Check sheet for the modelled part. Datum: model origin and axes. Units: mm. A direction names the side the tool comes from. Coordinates: 2 decimals unless noted, no trailing zeros. Loops run counter-clockwise (first coordinate to the right, second up) from the corner with the lowest first, then second, coordinate; pieces in that order, holes last. Notation, with made-up numbers: (9, 73.25) - (43, 73.25) arc R30 ccw to (43, 96.25) - close; hole circle Ø8 at (42, 73). An arc over 180 degrees is marked (long way). Use a Markdown table: item, result. Add a question column.
1) Tool access check on faces 4 (the flat face through (-9.5, -0.1, 19.2)), 5 (the cylindrical face through (-5.158, -3.955, 2.535)). Record the directions out of +Z, -Z, +X, -X, +Y, -Y that give a thin tool (end or side, any length) a straight path to the whole face; none if there is none.
2) Go/stop test with flat-tipped pins: P1, Ø6.5, axis at y = 1, z = 13.5, coming from the +X side; P2, Ø3.5, axis at x = 14, y = -6, coming from the -Z side. Record where each tip stops, or that it passes through.
3) Sectioned sample at A-A, the plane y = 6. Enter the section's corners in (x, z), then the cut area to 3 significant figures.
4) Draft check along Y on faces 1 (the cylindrical face through (-14, 0, 8)), 2 (the cylindrical face through (8.93, 0.13, 5.6)), 3 (the cylindrical face through (16.93, 8.9, 13.69)). Enter one of: pulls with the +Y half, pulls with the -Y half, needs draft (parallel to the pull), parting line crosses it, or undercut.
5) Sectioned sample at C-C, the plane x = 0. Enter the section's corners in (y, z), then the cut area to 3 significant figures.
6) Sectioned sample at B-B, the plane z = 18.5. Enter the section's corners in (x, y), then the cut area to 3 significant figures.
7) Thickness scan on line 1 (Y direction, x = 14, z = 20.75); line 2 (Y direction, x = -14, z = 10.5); line 3 (Y direction, x = -12, z = 13.5). Record the ranges inside material, lowest first.
8) Sectioned sample at D-D, the plane x = 10. Enter the section's corners in (y, z), then the cut area to 3 significant figures.
from build123d import *

# Parameters (mm, degrees)
SKETCH_1_W          = 35
SKETCH_1_H          = 19
SKETCH_1_R          = 1.5
EXTRUDE_1_DEPTH     = 27
SKETCH_2_W          = 19
SKETCH_2_H          = 17
CUT_EXTRUDE_1_DEPTH = 38.366428783
SKETCH_3_R          = 5.5
CUT_EXTRUDE_2_DEPTH = 46.213382975
SKETCH_4_R          = 6.5
CUT_EXTRUDE_3_DEPTH = 34.548472527
FILLET_1_R          = 2
FILLET_2_R          = 2


with BuildPart() as part:
    # 草图1 → 凸台-拉伸1 (new body)
    with BuildSketch(Plane.XY):
        Rectangle(SKETCH_1_W, SKETCH_1_H)
        with Locations((-14, 6)):
            Circle(SKETCH_1_R, mode=Mode.SUBTRACT)
        with Locations((14, 6)):
            Circle(SKETCH_1_R, mode=Mode.SUBTRACT)
        with Locations((14, -6)):
            Circle(SKETCH_1_R, mode=Mode.SUBTRACT)
        with Locations((-14, -6)):
            Circle(SKETCH_1_R, mode=Mode.SUBTRACT)
    extrude(amount=EXTRUDE_1_DEPTH)

    # 草图2 → 切除-拉伸1 (cut, through all)
    with BuildSketch(Plane.XZ.offset(9.5)):
        with Locations((0, 13.5)):
            Rectangle(SKETCH_2_W, SKETCH_2_H)
    extrude(amount=-CUT_EXTRUDE_1_DEPTH, mode=Mode.SUBTRACT)

    # 草图3 → 切除-拉伸2 (cut, through all)
    with BuildSketch(Plane.ZY.offset(17.5)):
        with Locations((13.5, 0)):
            Circle(SKETCH_3_R)
    extrude(amount=-CUT_EXTRUDE_2_DEPTH, mode=Mode.SUBTRACT)

    # 草图4 → 切除-拉伸3 (cut, through all)
    with BuildSketch(Plane.XY.offset(27)):
        Circle(SKETCH_4_R)
    extrude(amount=-CUT_EXTRUDE_3_DEPTH, mode=Mode.SUBTRACT)

    # 圆角1
    fillet_1_edges = [part.edges().sort_by_distance(p)[0] for p in [
        (9.5, 0, 22),
        (9.5, 0, 5),
        (-9.5, 0, 5),
        (-9.5, 0, 22),
    ]]
    fillet(fillet_1_edges, radius=FILLET_1_R)

    # 圆角2
    fillet_2_edges = [part.edges().sort_by_distance(p)[0] for p in [
        (17.5, -9.5, 13.5),
        (-17.5, -9.5, 13.5),
        (-17.5, 9.5, 13.5),
        (17.5, 9.5, 13.5),
    ]]
    fillet(fillet_2_edges, radius=FILLET_2_R)


solid = part.part
Solved:
| question | item | result |
|---|---|---|
| 1 | face 4 | +Y, -Y |
| 1 | face 5 | +Z, -Z |
| 2 | P1 | passes through |
| 2 | P2 | stops at z = 0 |
| 3 | outline | (-17.5, 0) - (-15.5, 0) - (-15.5, 27) - (-17.5, 27) - close; (-12.5, 0) - (-2.5, 0) - (-2.5, 5) - (-7.5, 5) arc R2 cw to (-9.5, 7) - (-9.5, 20) arc R2 cw to (-7.5, 22) - (-2.5, 22) - (-2.5, 27) - (-12.5, 27) - close; (2.5, 0) - (12.5, 0) - (12.5, 27) - (2.5, 27) - (2.5, 22) - (7.5, 22) arc R2 cw to (9.5, 20) - (9.5, 7) arc R2 cw to (7.5, 5) - (2.5, 5) - close; (15.5, 0) - (17.5, 0) - (17.5, 27) - (15.5, 27) - close |
| 3 | area | 413 mm2 |
| 4 | face 1 | undercut |
| 4 | face 2 | needs draft |
| 4 | face 3 | pulls with the +Y half |
| 5 | outline | (-9.5, 0) - (-6.5, 0) - (-6.5, 5) - (-9.5, 5) - close; (-9.5, 22) - (-6.5, 22) - (-6.5, 27) - (-9.5, 27) - close; (6.5, 0) - (9.5, 0) - (9.5, 5) - (6.5, 5) - close; (6.5, 22) - (9.5, 22) - (9.5, 27) - (6.5, 27) - close |
| 5 | area | 60.0 mm2 |
| 6 | outline | (-17.5, -7.5) arc R2 ccw to (-15.5, -9.5) - (-9.5, -9.5) - (-9.5, -2.29) - (-17.5, -2.29) - close; (-17.5, 2.29) - (-9.5, 2.29) - (-9.5, 9.5) - (-15.5, 9.5) arc R2 ccw to (-17.5, 7.5) - close; (9.5, -9.5) - (15.5, -9.5) arc R2 ccw to (17.5, -7.5) - (17.5, -2.29) - (9.5, -2.29) - close; (9.5, 2.29) - (17.5, 2.29) - (17.5, 7.5) arc R2 ccw to (15.5, 9.5) - (9.5, 9.5) - close; hole circle Ø3 at (-14, -6); hole circle Ø3 at (-14, 6); hole circle Ø3 at (14, -6); hole circle Ø3 at (14, 6) |
| 6 | area | 199 mm2 |
| 7 | line 1 | y = -9.5 to -7.5, -4.5 to 4.5, 7.5 to 9.5 |
| 7 | line 2 | y = -9.5 to -7.5, 7.5 to 9.5 |
| 7 | line 3 | y = -9.5 to -5.5, 5.5 to 9.5 |
| 8 | outline | (-9.5, 0) - (9.5, 0) - (9.5, 27) - (-9.5, 27) - close; hole circle Ø11 at (0, 13.5) |
| 8 | area | 418 mm2 |
